```python
from build123d import *

# Parameters (mm, degrees)
BOSS_EXTRUDE3_DEPTH        = 10
SKETCH4_R                  = 1.5
BOSS_EXTRUDE4_DEPTH        = 5
RIB6_REACH                 = 158.985
SKETCH5_WALL_W             = 329.861950248
SKETCH5_WALL_H             = 2.5
CHAMFER2_SIZE              = 1
CHAMFER3_SIZE              = 5.5
CHAMFER3_SIZE_2            = 9
LPATTERN4_COUNT            = 2
LPATTERN4_PITCH            = 75
LPATTERN4_COPY_1_REACH     = 158.985
LPATTERN4_COPY_1_SKETCH_W  = 329.861950248
LPATTERN4_COPY_1_SKETCH_H  = 2.5
CHAMFER2_OF_LPATTERN4_SIZE = 1
SKETCH8_R                  = 2.05
CUT_EXTRUDE1_DEPTH         = 4
SKETCH9_R                  = 1.6
CUT_EXTRUDE2_DEPTH         = 5


with BuildPart() as part:
    # Sketch2 → Boss-Extrude3 (new body)
    with BuildSketch(Plane(origin=(0, 0, 0), x_dir=(1, 0, 0), z_dir=(0, 1, 0))):
        with BuildLine():
            Line((-138.973021921, 39.179223473), (-139.022764358, 17.179279707))
            Line((-139.022764358, 17.179279707), (73.976691191, 16.697682479))
            Line((73.976691191, 16.697682479), (74.026978079, 38.697625014))
            Line((74.026978079, 38.697625014), (67.526578048, 38.712322585))
            Line((67.526578048, 38.712322585), (67.51414235, 33.212297518))
            Line((67.51414235, 33.212297518), (58.599731895, 33.232453229))
            ThreePointArc((58.599731895, 33.232453229), (42.488076808, 21.768891824), (26.428425, 33.305193378))
            Line((26.428425, 33.305193378), (17.51414235, 33.3253488))
            Line((17.51414235, 33.3253488), (17.526578048, 38.825373866))
            Line((17.526578048, 38.825373866), (-7.473230244, 38.881899074))
            Line((-7.473230244, 38.881899074), (-7.485665941, 33.381874007))
            Line((-7.485665941, 33.381874007), (-16.400076396, 33.402029717))
            ThreePointArc((-16.400076396, 33.402029717), (-32.511731484, 21.938468313), (-48.571383292, 33.474769867))
            Line((-48.571383292, 33.474769867), (-57.485665941, 33.494925288))
            Line((-57.485665941, 33.494925288), (-57.473230244, 38.994950355))
            Line((-57.473230244, 38.994950355), (-82.473038536, 39.051475562))
            Line((-82.473038536, 39.051475562), (-82.485474233, 33.551450496))
            Line((-82.485474233, 33.551450496), (-91.399884688, 33.571606206))
            ThreePointArc((-91.399884688, 33.571606206), (-107.511539776, 22.108044802), (-123.571191584, 33.644346356))
            Line((-123.571191584, 33.644346356), (-132.485474233, 33.664501777))
            Line((-132.485474233, 33.664501777), (-132.473038536, 39.164526844))
            Line((-132.473038536, 39.164526844), (-138.973021921, 39.179223473))
        make_face()
    extrude(amount=BOSS_EXTRUDE3_DEPTH)

    # Sketch4 → Boss-Extrude4 (add)
    with BuildSketch(Plane(origin=(0.087874316, 0, -38.864803222), x_dir=(-0.99999744389135, 0, -0.002261019850970016), z_dir=(0.002261019850970016, 0, -0.99999744389135))):
        Polygon((62.56118779, -12), (57.561251693, 0), (82.561123887, 0), (77.56118779, -12), align=None)
        with Locations((70.06118779, -8.5)):
            Circle(SKETCH4_R, mode=Mode.SUBTRACT)
    boss_extrude4 = extrude(amount=-BOSS_EXTRUDE4_DEPTH)

    # Sketch5 wall → Rib6 (add, up to next)
    with BuildSketch(Plane(origin=(-77.492333887, -6, -30.540192335), x_dir=(-0.001139262394, 0.863778900906, 0.503869737562), z_dir=(-0.001953021242, -0.503871025511, 0.863776692993)), mode=Mode.PRIVATE) as rib6_sk1:
        with Locations((0, -1.25)):
            Rectangle(SKETCH5_WALL_W, SKETCH5_WALL_H)
    rib6_tool1 = extrude(rib6_sk1.sketch, amount=-RIB6_REACH, mode=Mode.PRIVATE) - part.part
    rib6 = rib6_tool1.solids().sort_by_distance((-77.492333887, -6, -30.540192335))[0]
    add(rib6)

    # Mirror2: Rib6 across plane
    add(rib6.mirror(Plane(origin=(-70.061008706, 0, -0.158409736), x_dir=(-0.0022610198509701073, 0, 0.99999744389135), z_dir=(0.99999744389135, 0, 0.002261019850970107))))

    # Chamfer2
    chamfer2_edges = [part.edges().sort_by_distance(p)[0] for p in [
        (-68.484443323, -8.5, -34.01983421),
    ]]
    chamfer(chamfer2_edges, length=CHAMFER2_SIZE)

    # Chamfer3
    # the kernel refuses this chamfer: 9, 5.5 mm, written as the material it takes off along each edge
    with BuildSketch(Plane(origin=(-162.295390883, 0, -17.231899712), x_dir=(0.0022577295255832275, -0.053929224624231706, -0.9985422081158205), z_dir=(0.9999974438913499, 0, 0.0022610198509699707))) as chamfer3_piece_1:
        Polygon((CHAMFER3_SIZE * 0.998544760505, CHAMFER3_SIZE * 0.0539292246242), (-CHAMFER3_SIZE_2 * 0.0539292246242, CHAMFER3_SIZE_2 * 0.998544760505), (0, 0), align=None)
    extrude(amount=259.545372026, mode=Mode.SUBTRACT)

    # LPattern4: Boss-Extrude4, Rib6 ×2
    with Locations(*[Vector(0.9999974438913499, 0, 0.002261019850970079) * (i * LPATTERN4_PITCH) for i in range(1, LPATTERN4_COUNT)]):
        add(boss_extrude4)
        add(rib6)

    # LPattern4 copy 1 sketch → LPattern4 copy 1 (add, up to next)
    with BuildSketch(Plane(origin=(12.507436062, -6, -30.336700548), x_dir=(-0.0011392623880184954, 0.863778900906, 0.5038697375620136), z_dir=(-0.0019530212415939509, -0.503871025511, 0.863776692993001)), mode=Mode.PRIVATE) as lpattern4_copy_1_sk1:
        with Locations((0, 1.25)):
            Rectangle(LPATTERN4_COPY_1_SKETCH_W, LPATTERN4_COPY_1_SKETCH_H)
    lpattern4_copy_1_tool1 = extrude(lpattern4_copy_1_sk1.sketch, amount=-LPATTERN4_COPY_1_REACH, mode=Mode.PRIVATE) - part.part
    add(lpattern4_copy_1_tool1.solids().sort_by_distance((12.507436062, -6, -30.336700548))[0])

    # Chamfer2 of LPattern4
    chamfer2_of_lpattern4_edges = [part.edges().sort_by_distance(p)[0] for p in [
        (6.515364969, -8.5, -33.850257721),
    ]]
    chamfer(chamfer2_of_lpattern4_edges, length=CHAMFER2_OF_LPATTERN4_SIZE)

    # Sketch8 → Cut-Extrude1 (cut)
    with BuildSketch(Plane(origin=(0, 10, 0), x_dir=(1, 0, 0), z_dir=(0, 1, 0))):
        with Locations((-129.018242433, 19.156613217)):
            Circle(SKETCH8_R)
    cut_extrude1 = extrude(amount=-CUT_EXTRUDE1_DEPTH, mode=Mode.SUBTRACT)

    # Sketch9 → Cut-Extrude2 (cut)
    with BuildSketch(Plane(origin=(0, 6, 0), x_dir=(1, 0, 0), z_dir=(0, 1, 0))):
        with Locations((-129.018242433, 19.156613217)):
            Circle(SKETCH9_R)
    cut_extrude2 = extrude(amount=-CUT_EXTRUDE2_DEPTH, mode=Mode.SUBTRACT)

    # Mirror4: Cut-Extrude1, Cut-Extrude2 across plane
    add(cut_extrude1.mirror(Plane(origin=(-32.561168463, 0, -0.073621636), x_dir=(-0.002261019850969509, 0, 0.99999744389135), z_dir=(-0.99999744389135, 0, -0.0022610198509695084))), mode=Mode.SUBTRACT)
    add(cut_extrude2.mirror(Plane(origin=(-32.561168463, 0, -0.073621636), x_dir=(-0.002261019850969509, 0, 0.99999744389135), z_dir=(-0.99999744389135, 0, -0.0022610198509695084))), mode=Mode.SUBTRACT)


solid = part.part
```
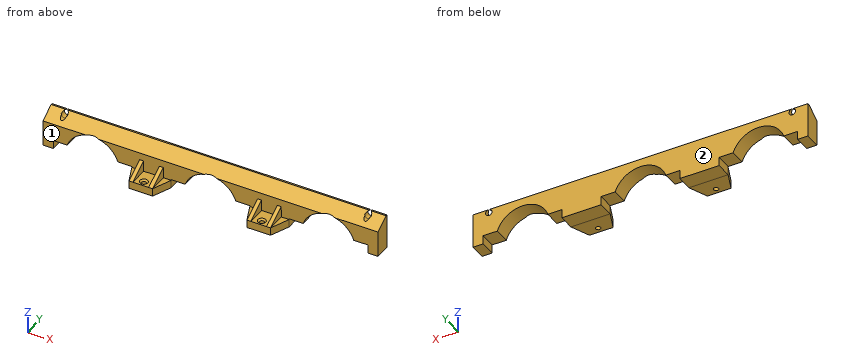
CAD build for the part. Positions are in the model's coordinates, mm. Face numbers are marked on the shaded views. A direction names the side the tool comes from. Coordinates: 2 decimals unless noted, no trailing zeros. Order: outer loops, then holes, each group sorted by start corner. A loop starts at its lowest first (then second) coordinate and runs counter-clockwise, first axis right, second up. Notation, with made-up numbers: (62.25, 87.5) - (109.25, 87.5) arc R16 cw to (109.25, 96.5) - close; hole circle Ø5 at (-18, 31). An arc over 180 degrees is marked (long way). Answer in a Markdown table with one row per item.
1. Flat gauge pins, fed straight in: P1, Ø5, axis at x = 63, z = -27.5, coming from the -Y side; P2, Ø5.5, axis at x = 63.98, z = -18.72, coming from the -Y side; P3, Ø3.5, axis at x = -129.02, z = -19.16, coming from the +Y side; P4, Ø8, axis at x = 44, y = -7, coming from the -Z side. Where does each tip first touch, or does it go through?
Answer:
| item | result |
|---|---|
| P1 | y = 0 |
| P2 | y = 1.23 |
| P3 | y = 6 |
| P4 | through |
2. 3-axis set-ups, long thin cutter, end or side, ignore diameter. For the marked faces 1 and 2: which of +Z, -Z, +X, -X, +Y, -Y reach the whole face in a straight line?
Answer:
| item | result |
|---|---|
| face 1 | +Z, -Z, -X, -Y |
| face 2 | +Z, -Z, +X, -X, +Y |
3. Slice it at A-A, the plane y = -2.5. List the corners of the cut face in (x, z).
Answer:
| item | result |
|---|---|
| outline | (-81.44, -34.05) - (-81.43, -39.05) - (-58.51, -39) - (-58.53, -34) - (-62.48, -34.01) - (-62.5, -28.46) - (-65, -28.47) - (-64.98, -34.01) - (-74.98, -34.03) - (-75, -28.49) - (-77.5, -28.5) - (-77.48, -34.04) - close; (-6.44, -33.88) - (-6.43, -38.88) - (16.48, -38.83) - (16.47, -33.83) - (12.52, -33.84) - (12.5, -28.3) - (10, -28.3) - (10.02, -33.84) - (0.02, -33.86) - (0, -28.32) - (-2.5, -28.33) - (-2.48, -33.87) - close |
4. Drill centre lines: L1, parallel to X at y = -3.25, z = -32.5; L2, parallel to X at y = 5.75, z = -31.75; L3, parallel to Y at x = -115.5, z = -23.75. Where is each one in solid material? Low to high. Write a range as from..to.
Answer:
| item | result |
|---|---|
| L1 | -77.49..-74.99, -64.99..-62.49, -2.49..0.01, 10.01..12.51 |
| L2 | -138.99..-122.8, -92.15..-47.88, -17.07..27.04, 58.01..74.01 |
| L3 | 0..10 |
5. Slice it at D-D, the plane x = 49. List the corners of the cut face in (y, z).
Answer:
| item | result |
|---|---|
| outline | (0, -23.05) - (10, -23.05) - (10, -16.75) - (9, -16.75) - (0, -22.25) - close |
6. Slice it at C-C, the plane x = -115. List the corners of the cut face in (y, z), then the cut area to 3 significant figures.
Answer:
| item | result |
|---|---|
| outline | (0, -23.87) - (10, -23.87) - (10, -17.12) - (9, -17.12) - (0, -22.62) - close |
| area | 42.7 mm² |
7. Slice it at B-B, the plane z = -30. Give the number of separate pieces and of enclosed holes in the cut face, then the cut area to 3 significant figures.
Answer:
| item | result |
|---|---|
| separate pieces | 4 |
| enclosed holes | 0 |
| area | 1,310 mm² |
